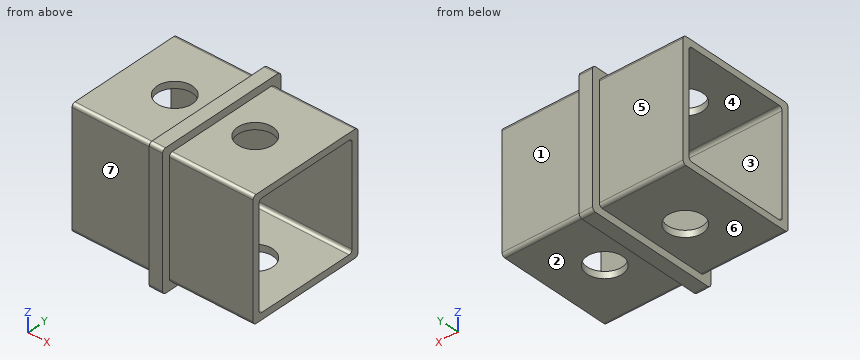
Autodesk Inventor part; units mm, degrees
ref_plane "YZ Plane" through (0, 0, 0) normal (1, 0, 0) x (0, 1, 0)
ref_plane "XZ Plane" through (0, 0, 0) normal (0, 1, 0) x (-1, 0, 0)
ref_plane "XY Plane" through (0, 0, 0) normal (0, 0, 1) x (1, 0, 0)
sketch "Skizze1" plane through (0, 0, 0) normal (1, 0, 0) x (0, 1, 0)
  line L0 (-16.75, 17.75) -> (16.75, 17.75)
  line L1 (17.75, 16.75) -> (17.75, -16.75)
  line L2 (16.75, -17.75) -> (-16.75, -17.75)
  line L3 (-17.75, -16.75) -> (-17.75, 16.75)
  line L4 (-17.75, 17.75) -> (17.75, -17.75) construction
  line L5 (17.75, 17.75) -> (-17.75, -17.75) construction
  line L6 (-14.75, 15.75) -> (14.75, 15.75)
  line L7 (15.75, 14.75) -> (15.75, -14.75)
  line L8 (14.75, -15.75) -> (-14.75, -15.75)
  line L9 (-15.75, -14.75) -> (-15.75, 14.75)
  line L10 (-15.75, 15.75) -> (15.75, -15.75) construction
  line L11 (15.75, 15.75) -> (-15.75, -15.75) construction
  arc A0 (17.75, 16.75) -> (16.75, 17.75) centre (16.75, 16.75) ccw
  arc A1 (-16.75, 17.75) -> (-17.75, 16.75) centre (-16.75, 16.75) ccw
  arc A2 (-17.75, -16.75) -> (-16.75, -17.75) centre (-16.75, -16.75) ccw
  arc A3 (16.75, -17.75) -> (17.75, -16.75) centre (16.75, -16.75) ccw
  arc A4 (14.75, -15.75) -> (15.75, -14.75) centre (14.75, -14.75) ccw
  arc A5 (-15.75, -14.75) -> (-14.75, -15.75) centre (-14.75, -14.75) ccw
  arc A6 (-14.75, 15.75) -> (-15.75, 14.75) centre (-14.75, 14.75) ccw
  arc A7 (15.75, 14.75) -> (14.75, 15.75) centre (14.75, 14.75) ccw
  point P0 (0, 0)
  dimension "d0" = 35.5
  dimension "d1" = 35.5
  dimension "d2" = 31.5
  dimension "d3" = 31.5
  dimension "d4" = 1
extrude "Extrusion1" add sketch "Skizze1" along normal blind 25
sketch "Skizze2" plane through (0, 0, 0) normal (-1, 0, 0) x (0, 0, 1)
  line L0 (19, 20) -> (-19, 20)
  line L1 (-20, 19) -> (-20, -19)
  line L2 (-19, -20) -> (19, -20)
  line L3 (20, -19) -> (20, 19)
  line L4 (20, 20) -> (-20, -20) construction
  line L5 (-20, 20) -> (20, -20) construction
  line L6 (16.75, 17.75) -> (-16.75, 17.75)
  line L7 (-17.75, 16.75) -> (-17.75, -16.75)
  line L8 (-16.75, -17.75) -> (16.75, -17.75)
  line L9 (17.75, -16.75) -> (17.75, 16.75)
  line L10 (17.75, 17.75) -> (-17.75, -17.75) construction
  line L11 (-17.75, 17.75) -> (17.75, -17.75) construction
  arc A0 (19, -20) -> (20, -19) centre (19, -19) ccw
  arc A1 (20, 19) -> (19, 20) centre (19, 19) ccw
  arc A2 (-19, 20) -> (-20, 19) centre (-19, 19) ccw
  arc A3 (-20, -19) -> (-19, -20) centre (-19, -19) ccw
  arc A4 (-17.75, -16.75) -> (-16.75, -17.75) centre (-16.75, -16.75) ccw
  arc A5 (-16.75, 17.75) -> (-17.75, 16.75) centre (-16.75, 16.75) ccw
  arc A6 (17.75, 16.75) -> (16.75, 17.75) centre (16.75, 16.75) ccw
  arc A7 (16.75, -17.75) -> (17.75, -16.75) centre (16.75, -16.75) ccw
  line L12 (-16.75, 17.75) -> (16.75, 17.75)
  line L13 (17.75, 16.75) -> (17.75, -16.75)
  line L14 (16.75, -17.75) -> (-16.75, -17.75)
  line L15 (-17.75, -16.75) -> (-17.75, 16.75)
  line L16 (-17.75, 17.75) -> (17.75, -17.75) construction
  line L17 (17.75, 17.75) -> (-17.75, -17.75) construction
  arc A8 (17.75, 16.75) -> (16.75, 17.75) centre (16.75, 16.75) ccw
  arc A9 (17.75, 16.75) -> (16.75, 17.75) centre (16.75, 16.75) ccw
  arc A10 (16.75, -17.75) -> (17.75, -16.75) centre (16.75, -16.75) ccw
  arc A11 (-16.75, 17.75) -> (-17.75, 16.75) centre (-16.75, 16.75) ccw
  arc A12 (-17.75, -16.75) -> (-16.75, -17.75) centre (-16.75, -16.75) ccw
  point P0 (0, 0)
  dimension "d7" = 40
  dimension "d8" = 40
  dimension "d9" = 1
  dimension "d10" = 1
  dimension "d11" = 1
extrude "Extrusion2" add sketch "Skizze2" along normal blind 4 contours A1 L3 A0 L2 A3 L1 A2 L0 | A6 L9 A7 L8 A4 L7 A5 L6
sketch "Skizze3" plane through (-4, 0, 0) normal (-1, 0, 0) x (0, 0, 1)
  line L0 (-14.75, 15.75) -> (14.75, 15.75)
  line L1 (15.75, 14.75) -> (15.75, -14.75)
  line L2 (14.75, -15.75) -> (-14.75, -15.75)
  line L3 (-15.75, -14.75) -> (-15.75, 14.75)
  line L4 (-15.75, 15.75) -> (15.75, -15.75) construction
  line L5 (15.75, 15.75) -> (-15.75, -15.75) construction
  arc A0 (15.75, 14.75) -> (14.75, 15.75) centre (14.75, 14.75) ccw
  arc A1 (-14.75, 15.75) -> (-15.75, 14.75) centre (-14.75, 14.75) ccw
  arc A2 (-15.75, -14.75) -> (-14.75, -15.75) centre (-14.75, -14.75) ccw
  arc A3 (14.75, -15.75) -> (15.75, -14.75) centre (14.75, -14.75) ccw
  point P0 (0, 0)
  dimension "d14" = 31.5
  dimension "d15" = 1
extrude "Extrusion3" cut sketch "Skizze3" against normal blind 4
sketch "Skizze4" plane through (-4, 0, 0) normal (-1, 0, 0) x (0, 0, 1)
  line L0 (-16.75, 17.75) -> (16.75, 17.75)
  line L1 (17.75, 16.75) -> (17.75, -16.75)
  line L2 (16.75, -17.75) -> (-16.75, -17.75)
  line L3 (-17.75, -16.75) -> (-17.75, 16.75)
  line L4 (-17.75, 17.75) -> (17.75, -17.75) construction
  line L5 (17.75, 17.75) -> (-17.75, -17.75) construction
  line L6 (-14.75, 15.75) -> (14.75, 15.75)
  line L7 (15.75, 14.75) -> (15.75, -14.75)
  line L8 (14.75, -15.75) -> (-14.75, -15.75)
  line L9 (-15.75, -14.75) -> (-15.75, 14.75)
  line L10 (-15.75, 15.75) -> (15.75, -15.75) construction
  line L11 (15.75, 15.75) -> (-15.75, -15.75) construction
  arc A0 (17.75, 16.75) -> (16.75, 17.75) centre (16.75, 16.75) ccw
  arc A1 (16.75, -17.75) -> (17.75, -16.75) centre (16.75, -16.75) ccw
  arc A2 (-17.75, -16.75) -> (-16.75, -17.75) centre (-16.75, -16.75) ccw
  arc A3 (-16.75, 17.75) -> (-17.75, 16.75) centre (-16.75, 16.75) ccw
  arc A4 (-14.75, 15.75) -> (-15.75, 14.75) centre (-14.75, 14.75) ccw
  arc A5 (15.75, 14.75) -> (14.75, 15.75) centre (14.75, 14.75) ccw
  arc A6 (14.75, -15.75) -> (15.75, -14.75) centre (14.75, -14.75) ccw
  arc A7 (-15.75, -14.75) -> (-14.75, -15.75) centre (-14.75, -14.75) ccw
  point P0 (0, 0)
  dimension "d18" = 1
extrude "Extrusion4" add sketch "Skizze4" along normal blind 25
sketch "Skizze5" plane through (25, -16.75, 17.75) normal (0, 0, 1) x (1, 0, 0)
  line L0 (-25, 16.75) -> (-15, 16.75)
  line L1 (-15, 16.75) -> (-39, 16.75)
  circle A0 centre (-15, 16.75) radius 5.25
  circle A1 centre (-39, 16.75) radius 5.25
  dimension "d21" = 10
  dimension "d22" = 24
  dimension "d23" = 10.5
  dimension "d24" = 10.5
extrude "Extrusion5" cut sketch "Skizze5" against normal blind 50
properties part number "Verbinder" material "Edelstahl, 440C"
Here's how the part is built. I have some questions about the finished solid (model axes, mm). Face numbers are marked on the shaded views. A direction names the side the tool comes from. Coordinates: 2 decimals unless noted, no trailing zeros. Order: outer loops, then holes, each group sorted by start corner. A loop starts at its lowest first (then second) coordinate and runs counter-clockwise, first axis right, second up.
Item 1: If we section it at B-B, the plane x = -14: List the corners of the cut face in (y, z) for me, then the cut area to 3 significant figures.
Response values:
outline: (-17.75, -16.75) arc R1 ccw to (-16.75, -17.75) - (-5.25, -17.75) - (-5.25, -15.75) - (-14.75, -15.75) arc R1 cw to (-15.75, -14.75) - (-15.75, 14.75) arc R1 cw to (-14.75, 15.75) - (-5.25, 15.75) - (-5.25, 17.75) - (-16.75, 17.75) arc R1 ccw to (-17.75, 16.75) - close; (5.25, -17.75) - (16.75, -17.75) arc R1 ccw to (17.75, -16.75) - (17.75, 16.75) arc R1 ccw to (16.75, 17.75) - (5.25, 17.75) - (5.25, 15.75) - (14.75, 15.75) arc R1 cw to (15.75, 14.75) - (15.75, -14.75) arc R1 cw to (14.75, -15.75) - (5.25, -15.75) - close
area: 226 mm2
Item 2: If we section it at A-A, the plane y = 0: Give the number of separate pieces and of enclosed holes in the cut face, then the cut area to 3 significant figures.
Response values:
separate pieces: 6
enclosed holes: 0
area: 150 mm2
Item 3: I'm going to push flat-ended pins straight in: pin 1 Ø9 at (x, y) = (-15, -6.5) entering from +Z; pin 2 Ø12.5 at (x, z) = (16, 7.5) entering from +Y; pin 3 Ø1.5 at (x, z) = (-13, 4) entering from -Y; pin 4 Ø20 at (x, y) = (-12, 6) entering from +Z. Where does each tip first touch, or does it pass through?
Response values:
pin 1: stops at z = 17.75
pin 2: stops at y = 17.75
pin 3: stops at y = -17.75
pin 4: stops at z = 20
Item 4: If we section it at C-C, the plane y = -11: List the corners of the cut face in (x, z) for me, then the cut area to 3 significant figures.
Response values:
outline: (-29, -17.75) - (-4, -17.75) - (-4, -20) - (0, -20) - (0, -17.75) - (25, -17.75) - (25, -15.75) - (-29, -15.75) - close; (-29, 15.75) - (25, 15.75) - (25, 17.75) - (0, 17.75) - (0, 20) - (-4, 20) - (-4, 17.75) - (-29, 17.75) - close
area: 234 mm2
Item 5: I need wall thicknesses on probe 1 along Z at (x, y) = (2.5, -4); probe 2 along Y at (x, z) = (10, 16.45). Which ranges of each line are inside material? Lowest first, please.
Response values:
probe 1: z = -17.75 to -15.75, 15.75 to 17.75
probe 2: y = -17.75 to -5.25, 5.25 to 17.75
Item 6: Thinking about a two-plate mould opening in Y: for the marked faces 1, 2 and 3, which applies, pulls with the +Y half, pulls with the -Y half, needs draft (parallel to the pull), parting line crosses it, or undercut?
Response values:
face 1: pulls with the +Y half
face 2: needs draft
face 3: undercut
Item 7: Which directions (+Z, -Z, +X, -X, +Y, -Y) give clear straight access to the entire face, cutting with the end or side of a thin tool? Please do the marked faces 4, 5, 6 and 7.
Response values:
face 4: +X, -X
face 5: +Z, -Z, -X, +Y
face 6: -Z, -X, +Y, -Y
face 7: +Z, -Z, -X, -Y
